The drawing under review shows one solid part. Ordinate dimensions are in mm from its lowest x, y, z. Coordinates: 2 decimals unless noted, no trailing zeros. Write each loop counter-clockwise with the first axis right and the second up, starting at its lowest first coordinate (ties: lowest second). Pieces come first, ordered by that corner, then holes. Notation, with made-up numbers: M 84.25,46.25 L 142.25,46.25 A28 cw 142.25,72.25 Z; hole C 80,-6.75 d10. An arc over 180 degrees is marked long. Write item = value, one per line.
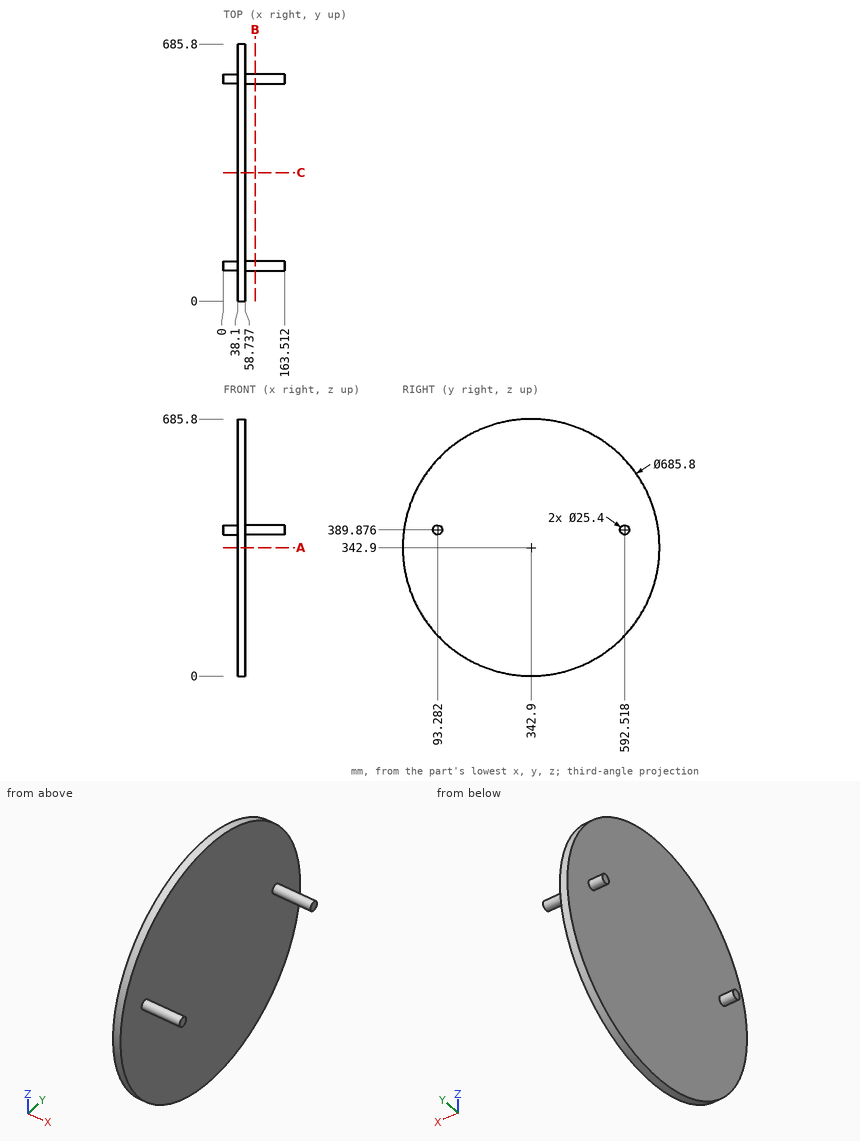
Q1. Consider section A-A, the plane z = 342.9. State the section outline as (x, y) points, and give its area (3 significant figures).
Check result:
outline = M 38.1,0 L 58.74,0 L 58.74,685.8 L 38.1,685.8 Z
area = 14,200 mm²
Q2. For P1, Ø3, axis at x = 54, y = 533, coming from the -Z side (1 decimal); P2, Ø1, axis at y = 115.5, z = 466.5, coming from the -X side; P3, Ø4, axis at x = 51, y = 255, coming from the -Z side, all flat-tipped, find the tip position at first contact; note any pin that passes through.
Check result:
P1 = 56.5
P2 = 38.1
P3 = 10.93
Q3. Consider section B-B, the plane x = 84.5. State the section outline as (y, z) points (1 decimal).
Check result:
outline = C 93.3,389.9 d25.4; C 592.5,389.9 d25.4
Q4. Wall thickness on line 1 (Y direction, x = 98, z = 388); line 2 (X direction, y = 247.5, z = 540); line 3 (Y direction, x = 47.5, z = 467.5): over which ranges is each line inside the solid? List them lowest first.
Check result:
line_1 = 80.72 to 105.84, 579.96 to 605.08
line_2 = 38.1 to 58.74
line_3 = 23.44 to 662.36
